Design review of the part built by this model. Coordinates are the model's own, in mm. Give positions to 0.01 mm unless a question says otherwise; leave off trailing zeros. Order: outer loops, then holes, each group sorted by start corner. A loop starts at its lowest first (then second) coordinate and runs counter-clockwise, first axis right, second up.
Autodesk Inventor part; units mm, degrees
ref_plane "Work Plane1" through (-17.0203, 16.0203, 0) normal (0, 1, 0) x (1, 0, 0)
ref_plane "YZ Plane" through (0, 0, 0) normal (1, 0, 0) x (0, 1, 0)
ref_plane "XZ Plane" through (0, 0, 0) normal (0, 1, 0) x (-1, 0, 0)
sketch "Sketch1" plane through (0, 0, 0) normal (0, 0, 1) x (1, 0, 0)
  circle A0 centre (16.0203, -16.0203) radius 2.75 construction
  circle A1 centre (-16.0203, 16.0203) radius 2.75 construction
  circle A2 centre (16.0203, 16.0203) radius 2.75 construction
  circle A3 centre (-16.0203, -16.0203) radius 2.75 construction
  circle A4 centre (0, 0) radius 12.5 construction
  line L0 (17.0203, -19.0203) -> (-17.0203, -19.0203)
  line L1 (-19.0203, -17.0203) -> (-19.0203, 17.0203)
  line L2 (-17.0203, 19.0203) -> (17.0203, 19.0203)
  line L3 (19.0203, 17.0203) -> (19.0203, -17.0203)
  line L4 (19.0203, -19.0203) -> (-19.0203, 19.0203) construction
  line L5 (-19.0203, -19.0203) -> (19.0203, 19.0203) construction
  arc A5 (-17.0203, 19.0203) -> (-19.0203, 17.0203) centre (-17.0203, 17.0203) ccw
  arc A6 (-19.0203, -17.0203) -> (-17.0203, -19.0203) centre (-17.0203, -17.0203) ccw
  arc A7 (17.0203, -19.0203) -> (19.0203, -17.0203) centre (17.0203, -17.0203) ccw
  arc A8 (19.0203, 17.0203) -> (17.0203, 19.0203) centre (17.0203, 17.0203) ccw
  circle A9 centre (0, 0) radius 14
  line L6 (16.9, 24.9006) -> (-16.9, 24.9006)
  line L7 (-16.9, 21.2821) -> (-16.9, 24.9006)
  line L8 (-21.2821, 16.9) -> (-16.9, 21.2821)
  line L9 (-24.9006, 16.9) -> (-21.2821, 16.9)
  line L10 (-24.9006, -16.9) -> (-24.9006, 16.9)
  line L11 (-21.2821, -16.9) -> (-24.9006, -16.9)
  line L12 (-16.9, -21.2821) -> (-21.2821, -16.9)
  line L13 (-16.9, -24.9006) -> (-16.9, -21.2821)
  line L14 (16.9, -24.9006) -> (-16.9, -24.9006)
  line L15 (16.9, -24.9006) -> (16.9, -21.2821)
  line L16 (16.9, -21.2821) -> (21.2821, -16.9)
  line L17 (21.2821, -16.9) -> (24.9006, -16.9)
  line L18 (24.9006, -16.9) -> (24.9006, -16.8)
  line L19 (24.9006, -16.8) -> (24.9006, 16.9)
  line L20 (24.9006, 16.9) -> (21.2821, 16.9)
  line L21 (21.2821, 16.9) -> (16.9, 21.2821)
  line L22 (16.9, 21.2821) -> (16.9, 24.9006)
  point P0 (16.8, 24.9006)
  point P1 (-16.8, 24.9006)
  point P2 (-24.9006, 16.8)
  point P3 (-24.9006, -16.8)
  point P4 (-16.8, -24.9006)
  point P5 (16.8, -24.9006)
  point P6 (24.9006, 16.8)
  dimension "d0" = 2
  dimension "d1" = 28
extrude "Extrusion1" add sketch "Sketch1" along normal blind 4 contours L0 A6 L1 A5 L2 A8 L3 A7
ref_plane "Work Plane1" through (-17.0203, 16.0203, 0) normal (0, 1, 0) x (1, 0, 0)
sketch "Sketch2" plane through (-17.0203, 16.0203, 0) normal (0, 1, 0) x (1, 0, 0)
  line L0 (3.0203, 0) -> (31.0203, 0) construction
  line L1 (0, 0) -> (-2, 0) construction
  line L2 (34.0406, 0) -> (0, 0) construction
  line L3 (36.0406, 0) -> (34.0406, 0) construction
  line L4 (34.0406, 0) -> (36.0406, 0) construction
  line L5 (0, 0) -> (34.0406, 0) construction
  line L6 (-2, 0) -> (0, 0) construction
  line L7 (31.0203, -4) -> (3.0203, -4) construction
  line L8 (-2, -4) -> (0, -4) construction
  line L9 (0, -4) -> (34.0406, -4) construction
  line L10 (34.0406, -4) -> (36.0406, -4) construction
  line L11 (36.0406, -4) -> (34.0406, -4) construction
  line L12 (34.0406, -4) -> (0, -4) construction
  line L13 (0, -4) -> (-2, -4) construction
  line L14 (33.8203, 0) -> (0.2203, 0) construction
  line L15 (33.0406, 0) -> (33.0406, -4) construction
  arc A0 (33.0406, -4.15) -> (33.0406, 1.15) centre (33.0406, -1.5) ccw
  line L16 (35.2252, -3) -> (36.2252, -4)
  line L17 (33.0406, -1.5) -> (35.6906, -1.5) construction
  line L18 (36.2252, -4) -> (33.0406, -4)
  line L19 (0, -4) -> (34.0406, -4) construction
  line L20 (33.0406, -4) -> (33.0406, 1.15)
  line L21 (36.0406, 0) -> (36.0406, -4)
  point P0 (17.0203, 0)
  dimension "d4" = 2.65
  dimension "d5" = 2.5
  dimension "d7" = 135
  dimension "d8" = 1.5
  dimension "d14" = 3
revolve "Revolution1" cut sketch "Sketch2" angle 360 about axis through (16.0203, 16.0203, 4) along (0, 0, -1)
pattern_circular "Circular Pattern1" count 4 over 360 about axis through (0, 0, -10) along (0, 0, 1) of "Revolution1"
properties part number "20_Cube_Insert_Sample_clamp_magnetic"
1. For line 1 along Y through (x, z) = (16, 1.65); line 2 along X through (y, z) = (-16, 1.3); line 3 along Y through (x, z) = (0, 2.25), list the stretches that pass through material, from the lowest coordinate up.
Recorded:
line 1: y = -19.02 to -18.67, -13.37 to 13.37, 18.67 to 19.02
line 2: x = -19.02 to -18.66, -13.38 to 13.38, 18.66 to 19.02
line 3: y = -19.02 to -14, 14 to 19.02
2. Take a section at C-C (z = 2.1). State the section outline as (x, y) points, then the cut area to 3 significant figures.
Recorded:
outline: (-19.02, -17.02) arc R2 ccw to (-17.02, -19.02) - (17.02, -19.02) arc R2 ccw to (19.02, -17.02) - (19.02, 17.02) arc R2 ccw to (17.02, 19.02) - (-17.02, 19.02) arc R2 ccw to (-19.02, 17.02) - close; hole circle Ø5.16 at (-16.02, -16.02); hole circle Ø5.16 at (-16.02, 16.02); hole circle Ø28 at (0, 0); hole circle Ø5.16 at (16.02, -16.02); hole circle Ø5.16 at (16.02, 16.02)
area: 744 mm2
3. For pin 1 (22.5 mm diameter, centred on x = 0, y = 0, fed in from -Z), flat-tipped, find the tip position at first contact; note if it passes through.
Recorded:
pin 1: passes through
4. Take a section at A-A (x = 0). State the section outline as (y, z) points, then the cut area to 3 significant figures.
Recorded:
outline: (-19.02, 0) - (-14, 0) - (-14, 4) - (-19.02, 4) - close; (14, 0) - (19.02, 0) - (19.02, 4) - (14, 4) - close
area: 40.2 mm2
5. Draft analysis for pull direction Y (two halves, no side actions). For faces 1 (the face through (0, -19.02, 2)), 2 (the face through (19.02, 0, 2)), 3 (the face through (12.932, 5.362, 1.972)), state which applies: pulls with the +Y half, pulls with the -Y half, needs draft (parallel to the pull), parting line crosses it, or undercut.
Recorded:
face 1: pulls with the -Y half
face 2: needs draft
face 3: undercut
